Part print with two shaded views. Sizes in mm from the minimum x, y, z corner. A direction names the side the tool comes from. Coordinates: 2 decimals unless noted, no trailing zeros. Write each loop counter-clockwise with the first axis right and the second up, starting at its lowest first coordinate (ties: lowest second). Pieces come first, ordered by that corner, then holes.
Q1. Band-saw the part on D-D, the plane z = 3.25. Write the cut outline in (x, y), plus the area to 3 significant figures.
Q2. Band-saw the part on C-C, the plane z = 1. Write the cut outline in (x, y), plus the area to 3 significant figures.
Q3. Band-saw the part on A-A, the plane x = 17.5. Write the cut outline in (y, z).
Q4. Which spindle directions (+Z, -Z, +X, -X, +Y, -Y) get a long thin tool onto all of the face, cutting with end or side? Do the marked faces 1 and 2. Say none if no direction does.
Q5. Pin check, flat tips, straight feed: P1, Ø1.5, axis at x = 25, y = 9.5, coming from the -Z side; P2, Ø4, axis at y = 20.5, z = 4.5, coming from the +X side; P3, Ø3.5, axis at x = 17.5, y = 17.5, coming from the +Z side; P4, Ø4, axis at x = 21.5, z = 5.5, coming from the +Y side. Stop position of each tip, or through.
Q6. Pull direction X, two halves, no side cores. Call the marked faces 3, 4 and 5: released by +X, released by -X, zero draft, split by the parting line, or undercut.
Q7. Drill centre lines: probe 1 along Y at (x, z) = (17.5, 2.85); probe 2 along Y at (x, z) = (17.5, 2.95); probe 3 along Z at (x, y) = (21, 5.5). Where is each one in solid material? Low to high.
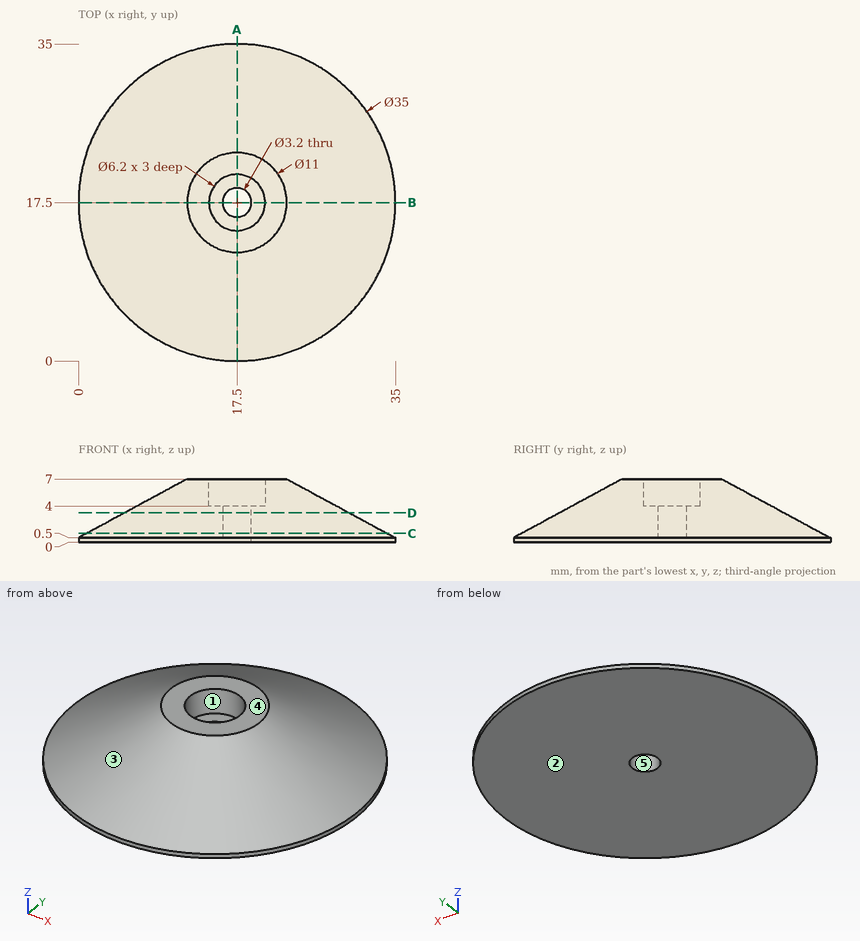
Answer sheet:
1. outline: circle Ø24.85 at (17.5, 17.5); hole circle Ø3.2 at (17.5, 17.5)
1. area: 477 mm2
2. outline: circle Ø33.15 at (17.5, 17.5); hole circle Ø3.2 at (17.5, 17.5)
2. area: 855 mm2
3. outline: (0, 0) - (15.9, 0) - (15.9, 4) - (14.4, 4) - (14.4, 7) - (12, 7) - (0, 0.5) - close; (19.1, 0) - (35, 0) - (35, 0.5) - (23, 7) - (20.6, 7) - (20.6, 4) - (19.1, 4) - close
4. face 1: +Z
4. face 2: -Z, +X, -X, +Y, -Y
5. P1: stops at z = 0
5. P2: stops at x = 31
5. P3: stops at z = 4
5. P4: stops at y = 28.83
6. face 3: split by the parting line
6. face 4: zero draft
6. face 5: undercut
7. probe 1: y = 4.34 to 15.9, 19.1 to 30.66
7. probe 2: y = 4.52 to 15.9, 19.1 to 30.48
7. probe 3: z = 0 to 3.21
